Can you work these out from the model? Positions are in its coordinate system, mm. A direction names the side the tool comes from. Give positions to 0.01 mm unless a question says otherwise; leave off trailing zeros. Write each loop counter-clockwise with the first axis right and the second up, starting at its lowest first coordinate (ties: lowest second). Pieces come first, ordered by that corner, then holes. Notation, with made-up numbers: (73, 49.25) -> (120, 49.25) arc R12 ccw to (120, 58.25) -> close; hole circle Ø3 at (37, 35). An arc over 180 degrees is marked (long way). Answer as CSV lines item,"result". Start each with the question number.
1. If we mould it in two halves opening along X, with no side actions, what happens to faces 1 (the face through (-24, 8.54, 1)), 2 (the face through (31.054, 2, 1)), 3 (the face through (21.639, 3.964, 0.783))? For each: pulls with the +X half, pulls with the -X half, needs draft (parallel to the pull), parting line crosses it, or undercut.
2. If we section it at B-B on z = 0.5: Count the separate pieces of the cut face and the enclosed holes in it, plus the area to 3 significant figures.
3. If we section it at C-C on y = 1.5: Write out the boundary of the cut face in (x, z).
4. If we section it at A-A on x = 24.5: Write out the boundary of the cut face in (y, z).
5. If we section it at D-D on x = -21: Write out the boundary of the cut face in (y, z), plus the area to 3 significant figures.
6. I need wall thicknesses on line 1 (Y direction, x = 20.5, z = 0.6); line 2 (Y direction, x = 25.5, z = 0.3); line 3 (Y direction, x = -5.5, z = 0.6). Which ranges of each line are inside material? Lowest first, please. Write a range as [from, to].
7. On a 3-axis mill with a long thin cutter (end or side, diameter ignored), from which of +Z, -Z, +X, -X, +Y, -Y can I reach the whole of each face in a straight line? I mean faces 4 (the face through (-24, -4.16, 1)), 5 (the face through (23, -4.16, 1)), 6 (the face through (23, 8.54, 1)). Say none if no direction works.
8. I'm going to push flat-ended pins straight in: P1, Ø6, axis at x = 23.57, y = 2.19, coming from the -Z side; P2, Ø0.5, axis at x = -25.5, z = 0.5, coming from the -Y side; P3, Ø0.5, axis at x = 23.5, z = 1, coming from the +Y side. Where does each tip first touch, or does it pass through?
```python
from build123d import *

# Parameters (mm, degrees)
SKETCH1_R           = 2.625
BOSS_EXTRUDE1_DEPTH = 1.5875
FILLET1_R           = 2.54


with BuildPart() as part:
    # Sketch1 → Boss-Extrude1 (new body)
    with BuildSketch(Plane(origin=(0, 0, 0), x_dir=(-1, 0, 0), z_dir=(0, 0, 1))):
        with BuildLine():
            Line((-16.092859192, 4.160440607), (-31.053947254, 4.160440607))
            Line((-31.053947254, 4.160440607), (-31.053947254, -8.539559393))
            Line((-31.053947254, -8.539559393), (-16.092859192, -8.539559393))
            ThreePointArc((-16.092859192, -8.539559393), (0.514545783, -19.969559393), (17.121950758, -8.539559393))
            Line((17.121950758, -8.539559393), (32.08303882, -8.539559393))
            Line((32.08303882, -8.539559393), (32.08303882, 4.160440607))
            Line((32.08303882, 4.160440607), (17.121950758, 4.160440607))
            ThreePointArc((17.121950758, 4.160440607), (0.514545783, 15.590440607), (-16.092859192, 4.160440607))
        make_face()
        with Locations(Location((-23.573403223, -2.189559393, 0), (0, 0, 180))):
            Circle(SKETCH1_R, mode=Mode.SUBTRACT)
        with Locations(Location((24.602494789, -2.189559393, 0), (0, 0, 180))):
            Circle(SKETCH1_R, mode=Mode.SUBTRACT)
    extrude(amount=BOSS_EXTRUDE1_DEPTH)

    # Fillet1
    fillet1_edges = [part.edges().sort_by_distance(p)[0] for p in [
        (-17.121950758, -4.160440607, 0.79375),
        (-32.08303882, -4.160440607, 0.79375),
        (-32.08303882, 8.539559393, 0.79375),
        (-17.121950758, 8.539559393, 0.79375),
        (16.092859192, 8.539559393, 0.79375),
        (31.053947254, 8.539559393, 0.79375),
        (31.053947254, -4.160440607, 0.79375),
        (16.092859192, -4.160440607, 0.79375),
    ]]
    fillet(fillet1_edges, radius=FILLET1_R)


solid = part.part
```
Computed values:
1,face 1,"needs draft"
1,face 2,"pulls with the +X half"
1,face 3,"undercut"
2,separate pieces,"1"
2,enclosed holes,"2"
2,area,"1,310 mm2"
3,outline,"(-32.08, 0) -> (-27.14, 0) -> (-27.14, 1.59) -> (-32.08, 1.59) -> close; (-22.07, 0) -> (21.04, 0) -> (21.04, 1.59) -> (-22.07, 1.59) -> close; (26.11, 0) -> (31.05, 0) -> (31.05, 1.59) -> (26.11, 1.59) -> close"
4,outline,"(-4.16, 0) -> (-0.27, 0) -> (-0.27, 1.59) -> (-4.16, 1.59) -> close; (4.65, 0) -> (8.54, 0) -> (8.54, 1.59) -> (4.65, 1.59) -> close"
5,outline,"(-4.16, 0) -> (8.54, 0) -> (8.54, 1.59) -> (-4.16, 1.59) -> close"
5,area,"20.2 mm2"
6,line 1,"y = [-4.16, 8.54]"
6,line 2,"y = [-4.16, 0.41], [3.97, 8.54]"
6,line 3,"y = [-14.88, 19.26]"
7,face 4,"+Z, -Z, -X, -Y"
7,face 5,"+Z, -Z, +X, -Y"
7,face 6,"+Z, -Z, +X, +Y"
8,P1,"stops at z = 0"
8,P2,"stops at y = -4.16"
8,P3,"stops at y = 8.54"
